The listing builds one solid part. Answer for the finished solid, in the listing's coordinates (mm). A direction names the side the tool comes from. Give positions to 0.01 mm unless a question says otherwise; leave off trailing zeros. Write each loop counter-clockwise with the first axis right and the second up, starting at its lowest first coordinate (ties: lowest second). Pieces come first, ordered by that corner, then holes. Notation, with made-up numbers: (56, 4) - (99, 4) arc R13 cw to (99, 10) - close; hole circle Ø5 at (62, -19). An arc over 180 degrees is marked (long way). Return JSON: item names as keys, results as strings.
from build123d import *

# Parameters (mm, degrees)
MAIN_FEATURES_W        = 2.1
MAIN_FEATURES_H        = 2.5
PEG_DEPTH              = 1.75
SKETCH1_3_W            = 25
SKETCH1_3_H            = 14.84
BLOCK_DEPTH            = 20
ROUNDED_PEG_EDGES_R    = 0.2
ROUNDED_BLOCK_EDGES_R  = 1
BREAK_PEG_EDGES_SIZE   = 0.1
BREAK_BLOCK_EDGES_SIZE = 1


with BuildPart() as part:
    # main_features → peg (new body)
    with BuildSketch(Plane.XY):
        with Locations((0, 12.44)):
            Rectangle(MAIN_FEATURES_W, MAIN_FEATURES_H)
    extrude(amount=-PEG_DEPTH)

    # Sketch1<3> → block (add)
    with BuildSketch(Plane.XY):
        with Locations((0, 7.62)):
            Rectangle(SKETCH1_3_W, SKETCH1_3_H)
    extrude(amount=BLOCK_DEPTH)

    # rounded_peg_edges
    rounded_peg_edges_edges = [part.edges().sort_by_distance(p)[0] for p in [
        (-1.05, 11.19, -0.875),
        (1.05, 11.19, -0.875),
        (1.05, 13.69, -0.875),
        (-1.05, 13.69, -0.875),
    ]]
    fillet(rounded_peg_edges_edges, radius=ROUNDED_PEG_EDGES_R)

    # rounded_block_edges
    rounded_block_edges_edges = [part.edges().sort_by_distance(p)[0] for p in [
        (-12.5, 0.2, 10),
        (12.5, 0.2, 10),
        (12.5, 15.04, 10),
        (-12.5, 15.04, 10),
    ]]
    fillet(rounded_block_edges_edges, radius=ROUNDED_BLOCK_EDGES_R)

    # break_peg_edges
    break_peg_edges_edges = [part.edges().sort_by_distance(p)[0] for p in [
        (0, 11.19, -1.75),
        (1.05, 12.44, -1.75),
        (0, 13.69, -1.75),
        (-1.05, 12.44, -1.75),
        (-0.991421356, 13.631421356, -1.75),
        (-0.991421356, 11.248578644, -1.75),
        (0.991421356, 13.631421356, -1.75),
        (0.991421356, 11.248578644, -1.75),
    ]]
    chamfer(break_peg_edges_edges, length=BREAK_PEG_EDGES_SIZE)

    # break_block_edges
    break_block_edges_edges = [part.edges().sort_by_distance(p)[0] for p in [
        (12.5, 7.62, 0),
        (12.5, 7.62, 20),
        (0, 0.2, 0),
        (-12.5, 7.62, 0),
        (0, 15.04, 0),
        (-12.207106781, 0.492893219, 0),
        (-12.207106781, 14.747106781, 0),
        (12.207106781, 14.747106781, 0),
        (12.207106781, 0.492893219, 0),
        (0, 0.2, 20),
        (0, 15.04, 20),
        (-12.5, 7.62, 20),
        (-12.207106781, 0.492893219, 20),
        (-12.207106781, 14.747106781, 20),
        (12.207106781, 14.747106781, 20),
        (12.207106781, 0.492893219, 20),
    ]]
    chamfer(break_block_edges_edges, length=BREAK_BLOCK_EDGES_SIZE)


solid = part.part
Item 1: A cutting plane is placed at B-B on x = 9. Determine the outline of the cut face in (y, z).
Answer below:
{"outline": "(0.2, 1) - (1.2, 0) - (14.04, 0) - (15.04, 1) - (15.04, 19) - (14.04, 20) - (1.2, 20) - (0.2, 19) - close"}
Item 2: A cutting plane is placed at A-A on y = 1.5. Determine the outline of the cut face in (x, z), then the cut area to 3 significant figures.
Answer below:
{"outline": "(-12.5, 1) - (-11.5, 0) - (11.5, 0) - (12.5, 1) - (12.5, 19) - (11.5, 20) - (-11.5, 20) - (-12.5, 19) - close", "area": "498 mm²"}
Item 3: For faces 1 (the face through (0, 11.19, -1)), 2 (the face through (1.05, 12, -1)), 3 (the face through (11.862, 14.395, 0.507)), 4 (the face through (0, 13.69, -1)), determine the directions among +Z, -Z, +X, -X, +Y, -Y from which every point of the face is accessible in a straight line to the end or side of a thin tool.
Answer below:
{"face 1": "-Z, +X, -X, -Y", "face 2": "-Z, +X, +Y, -Y", "face 3": "-Z, +X, +Y", "face 4": "-Z, +X, -X, +Y"}
Item 4: Flat-ended cylindrical pins translate along their axes: P1, Ø0.5, axis at x = -0.5, z = -0.5, coming from the +Y side; P2, Ø1.5, axis at x = -4.5, y = 6.5, coming from the -Z side; P3, Ø0.8, axis at y = 12.5, z = -1, coming from the -X side. Find the tip coordinate at first contact, or state that the pin passes through.
Answer below:
{"P1": "stops at y = 13.69", "P2": "stops at z = 0", "P3": "stops at x = -1.05"}
Item 5: Consider L1, parallel to Z at x = 8.25, y = 14; L2, parallel to X at y = 1, z = 9.5; L3, parallel to Z at x = 2, y = 14.5. Determine where each line is inside the solid, lowest interval first.
Answer below:
{"L1": "z = 0 to 20", "L2": "x = -12.48 to 12.48", "L3": "z = 0.46 to 19.54"}
